Verification items for the finished model (mm, model axes). Face numbers are marked on the shaded views. A direction names the side the tool comes from. Coordinates: 2 decimals unless noted, no trailing zeros. Write each loop counter-clockwise with the first axis right and the second up, starting at its lowest first coordinate (ties: lowest second). Pieces come first, ordered by that corner, then holes. Notation, with made-up numbers: (81, 22.25) -> (118, 22.25) arc R9 ccw to (118, 29.25) -> close; hole circle Ø7 at (77, 78.5). An arc over 180 degrees is marked (long way). Answer in a Markdown table with one row per item.
```python
from build123d import *

# Parameters (mm, degrees)
F0_R      = 21.4215
F1_DEPTH  = 10.2
F3_DEPTH  = 8.2
F4_R      = 12.24
F5_DEPTH  = 5.344
F6_W      = 8.2
F6_H      = 6
F7_DEPTH  = 25
F8_R      = 1
F9_R      = 10
F10_DEPTH = 6


with BuildPart() as f1:
    # F0 (on Right) → F1 (new body)
    with BuildSketch(Plane.YZ):
        Circle(F0_R)
    extrude(amount=-F1_DEPTH)

    # F2 (on face) → F3 (cut)
    with BuildSketch(Plane.YZ):
        with BuildLine():
            ThreePointArc((19.3182468731, -2), (-19.4215, 0), (19.3182468731, 2))
            Line((19.3182468731, 2), (21.3279315043, 2))
            ThreePointArc((21.3279315043, 2), (-21.4215, 0), (21.3279315043, -2))
            Line((21.3279315043, -2), (19.3182468731, -2))
        make_face()
    extrude(amount=-F3_DEPTH, mode=Mode.SUBTRACT)

    # F4 (on face) → F5 (cut)
    with BuildSketch(Plane(origin=(-10.2, 0, 0), x_dir=(0, -1, 0), z_dir=(-1, 0, 0))):
        Circle(F4_R)
    extrude(amount=-F5_DEPTH, mode=Mode.SUBTRACT)

    # F6 (on Top) → F7 (cut)
    with BuildSketch(Plane.XY):
        with Locations((-4.1, 0)):
            Rectangle(F6_W, F6_H)
    extrude(amount=F7_DEPTH, mode=Mode.SUBTRACT)

    # F8
    f8_edges = [f1.edges().sort_by_distance(p)[0] for p in [
        (-4.856, 3, 5.93333),
        (-4.856, -3, 5.93333),
        (-8.2, 0, 12.24),
    ]]
    fillet(f8_edges, radius=F8_R)

    # F9 (on face) → F10 (cut)
    with BuildSketch(Plane.YZ):
        Circle(F9_R)
    extrude(amount=-F10_DEPTH, mode=Mode.SUBTRACT)


solid = f1.part
```
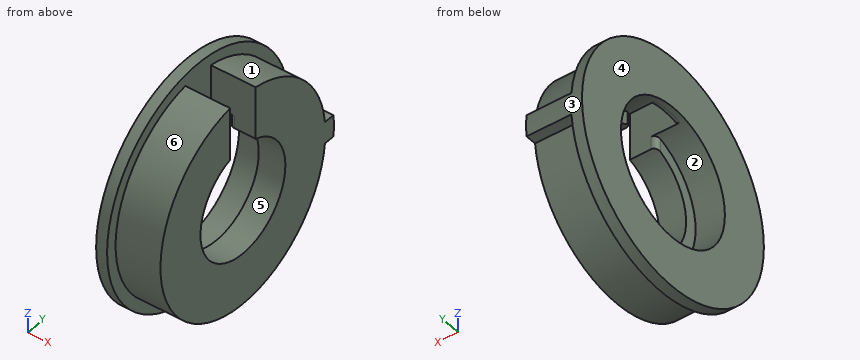
1. Sectioned sample at A-A, the plane y = 0. Record the cut outline in (x, z).
Findings below:
| item | result |
|---|---|
| outline | (-10.2, -21.42) -> (-8.2, -21.42) -> (-8.2, -19.42) -> (0, -19.42) -> (0, -10) -> (-4.86, -10) -> (-4.86, -12.24) -> (-10.2, -12.24) -> close; (-10.2, 12.24) -> (-9.2, 12.24) arc R1 ccw to (-8.2, 13.24) -> (-8.2, 21.42) -> (-10.2, 21.42) -> close |
2. Go/stop test with flat-tipped pins: pin 1 (4 mm diameter, centred on x = -7, y = 9.5, fed in from +Z); pin 2 (2 mm diameter, centred on y = -8.5, z = -11.5, fed in from +X); pin 3 (12 mm diameter, centred on y = 2.5, z = 2.5, fed in from -X); pin 4 (1 mm diameter, centred on x = -5.5, z = 5.5, fed in from -Y). Record where each tip stops, or that it passes through.
Findings below:
| item | result |
|---|---|
| pin 1 | stops at z = 19.91 |
| pin 2 | stops at x = 0 |
| pin 3 | passes through |
| pin 4 | stops at y = -18.77 |
3. Sectioned sample at B-B, the plane z = 0. Record the cut outline in (x, y), and give its area (3 significant figures).
Findings below:
| item | result |
|---|---|
| outline | (-10.2, -21.42) -> (-8.2, -21.42) -> (-8.2, -19.42) -> (0, -19.42) -> (0, -10) -> (-4.86, -10) -> (-4.86, -12.24) -> (-10.2, -12.24) -> close; (-10.2, 12.24) -> (-4.86, 12.24) -> (-4.86, 10) -> (0, 10) -> (0, 21.42) -> (-10.2, 21.42) -> close |
| area | 193 mm² |
4. Release check for a two-part mould opening along Y. For the marked faces 1, 2, 3 and 4 record: released by +Y, released by -Y, zero draft, split by the parting line, or undercut.
Findings below:
| item | result |
|---|---|
| face 1 | released by +Y |
| face 2 | undercut |
| face 3 | split by the parting line |
| face 4 | zero draft |
5. Material ranges on probe 1 along Y at (x, z) = (-1.1, 0); probe 2 along Y at (x, z) = (-1.25, -7); probe 3 along Z at (x, y) = (-2.5, 0), recorded low to high. Write a range as from..to.
Findings below:
| item | result |
|---|---|
| probe 1 | y = -19.42..-10, 10..21.42 |
| probe 2 | y = -18.12..-7.14, 7.14..18.12 |
| probe 3 | z = -19.42..-10 |
6. Access from +Z, -Z, +X, -X, +Y, -Y to the whole of each face (thin tool, end or side, straight path). Record for the marked faces 5 and 6.
Findings below:
| item | result |
|---|---|
| face 5 | +X, -X |
| face 6 | +X |
7. Sectioned sample at C-C, the plane z = -18. Record the cut outline in (x, y).
Findings below:
| item | result |
|---|---|
| outline | (-10.2, -11.61) -> (-8.2, -11.61) -> (-8.2, -7.29) -> (0, -7.29) -> (0, 7.29) -> (-8.2, 7.29) -> (-8.2, 11.61) -> (-10.2, 11.61) -> close |
